Solid Edge part; units mm, degrees
sketch "Sketch1" plane through (0, 0, 0) normal (0, 0, 1) x (1, 0, 0)
  line L0 (8.5, 15) -> (8.5, 12.9641)
  line L1 (8.5, 12.9641) -> (10.5, 13.5)
  line L2 (10.5, 13.5) -> (10.5, 10)
  line L3 (10.5, 10) -> (18.7929, 10)
  line L4 (18.7929, 10) -> (19.5, 10.7071)
  line L5 (19.5, 10.7071) -> (19.5, 14.6464)
  line L6 (19.5, 14.6464) -> (19.1464, 15)
  line L7 (19.1464, 15) -> (8.5, 15)
revolve "RevolvedProtrusion1" add sketch "Sketch1" angle 360 about axis through (10.5, 0, 0) along (-1, 0, 0)
hole "Bohrung_1" at (15.7, 15, 0) direction (0, -1, 0) diameter 5 depth 5.8175 countersink diameter 5.8 countersink angle 90
hole "Bohrung_2" at (15.7, 0, 9.298) direction (0, 0, 1) diameter 4 depth 5.702
sketch "Sketch2" plane through (15.7, 0, 0) normal (1, 0, 0) x (0, 1, 0)
  line L0 (16, 0) -> (16, -2.0095)
  line L1 (16, -2.0095) -> (15.5095, -2.5)
  line L2 (15.5095, -2.5) -> (10.75, -2.5)
  line L3 (10.75, -2.5) -> (10, -1.75)
  line L4 (10, -1.75) -> (10, 0)
  line L5 (10, 0) -> (16, 0)
revolve "RevolvedProtrusion2" add sketch "Sketch2" angle 360 about axis through (15.7, 10, 0) along (0, 1, 0)
cosmetic_thread "Thread1"
sketch "Sketch3" plane through (15.7, 16, 0) normal (0, 1, 0) x (-1, 0, 0)
  line L0 (-0.7217, 1.25) -> (-1.4434, 0)
  line L1 (-1.4434, 0) -> (-0.7217, -1.25)
  line L2 (-0.7217, -1.25) -> (0.7217, -1.25)
  line L3 (0.7217, -1.25) -> (1.4434, 0)
  line L4 (1.4434, 0) -> (0.7217, 1.25)
  line L5 (0.7217, 1.25) -> (-0.7217, 1.25)
extrude "Extrusionsausschnitt_1" cut sketch "Sketch3" against normal blind 2
properties part number "62599720_3"
Could you check a few things on this model? Use its own coordinates, in mm. A direction names the side the tool comes from. Coordinates: 2 decimals unless noted, no trailing zeros. Order: outer loops, then holes, each group sorted by start corner. A loop starts at its lowest first (then second) coordinate and runs counter-clockwise, first axis right, second up. Notation, with made-up numbers: M -38.5,-31 L -17.5,-31 A12 ccw -17.5,-8 Z; hole C -1.75,67 d5. An arc over 180 degrees is marked long. Use a Markdown table: item, result. Add a question column.
Q1. I want a section at A-A on y = 0. List the corners of the cut face in (x, z) for me, then the cut area to 3 significant figures.
Q2. We'd pull the mould along Z, two halves only. Please class faces 4 (the cylindrical face through (14, -12, 9)), 5 (the flat face through (14.62, 15.01, -0.63)), 6 (the flat face through (8.5, -9, -10)): pulls with the +Z half, pulls with the -Z half, needs draft (parallel to the pull), parting line crosses it, or undercut.
Q3. If I drill on L1, parallel to X at y = 0, z = 12; L2, parallel to Z at x = 13.5, y = 0; L3, parallel to Y at x = 15.5, z = 0, over which ranges is the centre line in solid material (lowest first)?
Q4. I want a section at B-B on x = 15.7. List the corners of the cut face in (y, z) for me.
Q5. I'm going to push flat-ended pins straight in: pin 1 (4 mm diameter, centred on x = 13, y = 6.5, fed in from -Z); pin 2 (1 mm diameter, centred on x = 10, y = -6, fed in from +Z); pin 3 (18 mm diameter, centred on y = 0, z = 0, fed in from +X); pin 4 (1 mm diameter, centred on x = 13, y = -2.5, fed in from -Z). Where does each tip first touch, or does it pass through?
Q6. Which directions (+Z, -Z, +X, -X, +Y, -Y) give clear straight access to the entire face, cutting with the end or side of a thin tool? Please do faces 1 (the cylindrical face through (17.652, -0.434, 12.435)), 2 (the flat face through (16, 15, -1.25)), 3 (the flat face through (10.5, -9, 5)).
Checked values:
| question | item | result |
|---|---|---|
| 1 | outline | M 8.5,-15 L 19.15,-15 L 19.5,-14.65 L 19.5,-10.71 L 18.79,-10 L 10.5,-10 L 10.5,-13.5 L 8.5,-12.96 Z; M 8.5,12.96 L 10.5,13.5 L 10.5,10 L 13.7,10 L 13.7,15 L 8.5,15 Z; M 17.7,10 L 18.79,10 L 19.5,10.71 L 19.5,14.65 L 19.15,15 L 17.7,15 Z |
| 1 | area | 76.4 mm² |
| 2 | face 4 | parting line crosses it |
| 2 | face 5 | undercut |
| 2 | face 6 | needs draft |
| 3 | L1 | 10.5 to 13.7, 17.7 to 19.5 |
| 3 | L2 | -15 to -10, 10 to 15 |
| 3 | L3 | -15 to -10, 10 to 14 |
| 4 | outline | M -2,9.8 L -2,14.87 A15 ccw long 14.76,-2.66 L 14.6,-2.5 L 15.51,-2.5 L 16,-2.01 L 16,-1.25 L 14,-1.25 L 14,1.25 L 16,1.25 L 16,2.01 L 15.51,2.5 L 14.6,2.5 L 14.76,2.66 A15 ccw 2,14.87 L 2,9.8 A10 cw 9.68,2.5 L 10.75,2.5 L 10,1.75 L 10,-1.75 L 10.75,-2.5 L 9.68,-2.5 A10 cw long Z |
| 5 | pin 1 | z = -14.31 |
| 5 | pin 2 | z = 13.96 |
| 5 | pin 3 | through |
| 5 | pin 4 | z = -14.87 |
| 6 | face 1 | +Z |
| 6 | face 2 | +Y |
| 6 | face 3 | none |
